Source: CAD feature listing. Evaluate the final solid. Frame: model axes, mm. Face numbers are marked on the shaded views. A direction names the side the tool comes from. Coordinates: 2 decimals unless noted, no trailing zeros. Order: outer loops, then holes, each group sorted by start corner. A loop starts at its lowest first (then second) coordinate and runs counter-clockwise, first axis right, second up.
Autodesk Inventor part; units mm, degrees
ref_plane "YZ Plane" through (0, 0, 0) normal (1, 0, 0) x (0, 1, 0)
ref_plane "XZ Plane" through (0, 0, 0) normal (0, 1, 0) x (-1, 0, 0)
ref_plane "XY Plane" through (0, 0, 0) normal (0, 0, 1) x (1, 0, 0)
sketch "Boceto1" plane through (0, 0, 0) normal (0, 1, 0) x (-1, 0, 0)
  line L0 (80, 47.68) -> (80, 52.68)
  line L1 (80, 47.68) -> (80, 22.68)
  line L2 (80, 22.68) -> (75, 22.68)
  line L3 (75, 22.68) -> (71.4886, 22.68)
  line L4 (80, 80) -> (80, 52.68)
  line L5 (20, 72.2842) -> (-29.4975, 121.7816)
  line L6 (20, 72.2842) -> (90, 72.2842) construction
  line L7 (-29.4975, 121.7816) -> (-22.4264, 128.8527)
  line L8 (29.9618, 80) -> (80, 80)
  arc A0 (71.4886, 22.68) -> (20, 72.2842) centre (0, 0) ccw
  line L9 (-22.4264, 128.8527) -> (26.4263, 80)
  line L10 (26.4263, 80) -> (29.9618, 80)
  dimension "d4" = 5
  dimension "d5" = 25
  dimension "d21" = 70
  dimension "d22" = 135
  dimension "d23" = 10
extrude "Extrusión5" add sketch "Boceto1" along normal blind 20
fillet "Empalme3" radius 80 1 edges at (-20, 10, 72.2842)
fillet "Empalme4" radius 3 4 edges at (29.4975, 10, 121.7816) (22.4264, 10, 128.8527) (-71.4886, 10, 22.68) (-80, 10, 22.68)
fillet "Empalme5" radius 30 1 edges at (-80, 10, 80)
chamfer "Chaflán1" distance 20 angle 45 1 edges at (-26.4263, 10, 80)
sketch "Boceto4" plane through (0, 20, 0) normal (0, 1, 0) x (1, 0, 0)
  arc A0 (-69.282, -40) -> (-27.3616, -75.1754) centre (0, 0) ccw
  line L0 (0, 0) -> (-69.282, -40) construction
  line L1 (0, 0) -> (80, 0) construction
  line L2 (0, 0) -> (-27.3616, -75.1754) construction
  line L3 (-69.282, -40) -> (-74.282, -40)
  line L4 (-74.282, -40) -> (-74.282, -47)
  arc A1 (-74.282, -47) -> (-27.3616, -75.1754) centre (-35.8026, -36.0762) ccw
  dimension "d35" = 80
  dimension "d36" = 150
  dimension "d37" = 40
  dimension "d38" = 5
  dimension "d39" = 7
  dimension "d40" = 40
extrude "Extrusión6" cut sketch "Boceto4" against normal blind 20
sketch "Boceto5" plane through (0, 20, 0) normal (0, 1, 0) x (1, 0, 0)
  line L0 (-80, -50) -> (-80, -25.68)
  line L1 (-46.4263, -80) -> (-50, -80)
  arc A0 (-80, -50) -> (-46.4263, -80) centre (-41.1827, -40.3452) ccw
  arc A1 (-80, -50) -> (-46.4263, -80) centre (-50.0008, -50.2137) ccw
  line L2 (-27.3616, -75.1754) -> (-17.3616, -75.1754) construction
  point P0 (0, 0)
  dimension "d43" = 40
  dimension "d44" = 30
extrude "Extrusión7" cut sketch "Boceto5" against normal blind 20
sketch "Boceto6" plane through (0, 20, 0) normal (0, 1, 0) x (1, 0, 0)
  line L0 (-36.5264, -71.1746) -> (-40.1604, -76.8501)
  line L1 (-40.1604, -76.8501) -> (-29.2954, -83.1239)
  line L2 (-29.2954, -83.1239) -> (-25.1938, -76.0206)
  line L3 (-25.1938, -76.0206) -> (-24.7057, -75.1754)
  line L4 (-24.7057, -75.1754) -> (-35.8148, -69.3243)
  line L5 (-35.8148, -69.3243) -> (-36.5264, -71.1746)
  point P0 (0, 0)
  point P1 (-74.282, -47)
  dimension "d50" = 44.8319
extrude "Extrusión8" add sketch "Boceto6" against normal blind 20
sketch "Boceto7" plane through (0, 20, 0) normal (0, 1, 0) x (1, 0, 0)
  arc A0 (-69.282, -40) -> (-36.5264, -71.1746) centre (0, 0) ccw
  line L0 (-69.282, -40) -> (-74.282, -40)
  line L1 (-69.282, -40) -> (-69.282, -40)
  arc A1 (-74.282, -47) -> (-39.5521, -75.9) centre (-35.8026, -36.0762) ccw
  line L2 (-55.1527, -57.9498) -> (-58.6667, -54.3895)
  line L3 (-66.0968, -62.1963) -> (-58.6667, -54.3895)
  line L4 (-62.599, -65.7738) -> (-55.1527, -57.9498)
  line L5 (-66.0968, -62.1963) -> (-67.4453, -63.6132)
  line L6 (-67.4453, -63.6132) -> (-64.0789, -67.3287)
  line L7 (-64.0789, -67.3287) -> (-62.599, -65.7738)
extrude "Extrusión9" add sketch "Boceto7" against normal blind 20 contours A0 L4 A1 L3 | A1 L7 L6 L5
sketch "Boceto8" plane through (-80, 0, 25.68) normal (-1, 0, 0) x (0, 0, 1)
  point P0 (-25.68, 0)
sketch "Boceto9" plane through (-80, 0, 25.68) normal (-1, 0, 0) x (0, 0, 1)
  line L0 (0, 20) -> (24.32, 20)
  line L1 (0, 0) -> (0, 20)
  line L2 (24.32, 20) -> (24.32, 0)
  line L3 (-3, 20) -> (0, 20)
  line L4 (12.16, 10) -> (22.16, 10) construction
  line L5 (19.2311, 17.0711) -> (20.9988, 15.3033)
  line L6 (19.2311, 17.0711) -> (17.4633, 18.8388)
  line L7 (5.0889, 2.9289) -> (6.8567, 1.1612)
  line L8 (5.0889, 2.9289) -> (3.3212, 4.6967)
  line L9 (3.3212, 4.6967) -> (17.4633, 18.8388)
  line L10 (20.9988, 15.3033) -> (6.8567, 1.1612)
  point P0 (-25.68, 0)
  dimension "d56" = 10
  dimension "d58" = 10
  dimension "d59" = 2.5
  dimension "d60" = 2.5
extrude "Extrusión10" add sketch "Boceto9" along normal blind 13
sketch "Boceto10" plane through (-80, 4.6967, 29.0012) normal (0, 0.7071, -0.7071) x (-1, 0, 0)
  line L0 (13, 0) -> (13, 20)
  line L1 (13, 20) -> (13, 0)
  line L2 (10, 10) -> (10, 15)
  line L3 (10, 15) -> (3, 15)
  line L4 (3, 15) -> (3, 5)
  line L5 (3, 5) -> (10, 5)
  line L6 (10, 5) -> (10, 10)
  point P0 (-80, -23.828)
  dimension "d64" = 5
  dimension "d65" = 7
  dimension "d66" = 10
extrude "Extrusión11" cut sketch "Boceto10" against normal blind 13
properties part number "Positioner_Adapter_Izq" material "ABS Plastic Black"
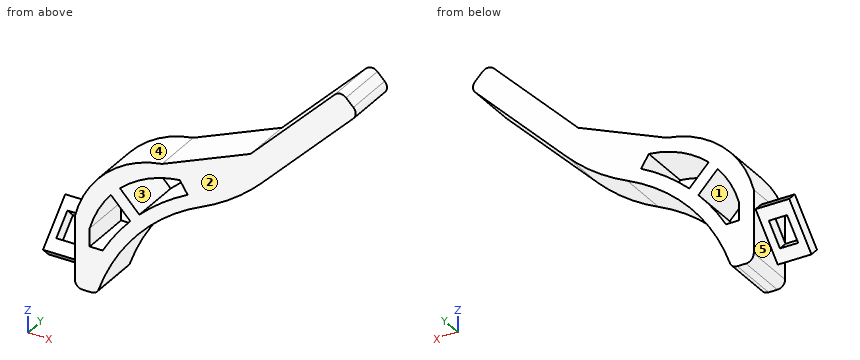
Q1. Pin query (flat end, axial travel): P1, Ø12, axis at x = -42, y = 13.5, coming from the -Z side; P2, Ø2.5, axis at x = -73, y = 5, coming from the +Z side; P3, Ø2, axis at y = 6, z = 43.5, coming from the +X side. Return the tip coordinate at first contact, or that it passes through.
Solutions:
P1: stops at z = 57.63
P2: stops at z = 66.15
P3: stops at x = -60.37
Q2. Material intervals for line 1 along Z through (x, y) = (-40.5, 7.5); line 2 along X through (y, z) = (8.5, 52); line 3 along X through (y, z) = (4.75, 57), sorted ascending.
Solutions:
line 1: z = 63.12 to 68.99, 75.8 to 82.45
line 2: x = -79.45 to -72.5, -60.79 to -54.05
line 3: x = -77.55 to -69.89, -61.15 to -48.74
Q3. Section query C-C on z = 101. Output: boundary loops of the cut face in (x, y), plus the area to 3 significant figures.
Solutions:
outline: (-5.43, 0) - (8.72, 0) - (8.72, 20) - (-5.43, 20) - close
area: 283 mm2
Q4. Section query A-A on x = -64. Output: boundary loops of the cut face in (y, z).
Solutions:
outline: (0, 39.1) - (20, 39.1) - (20, 48) - (0, 48) - close; (0, 59.99) - (20, 59.99) - (20, 73.2) - (0, 73.2) - close
Q5. Set-up query: the marked faces 1 and 2. Return all of +Z, -Z, +X, -X, +Y, -Y with unobstructed straight access to the full face (end or side cutting, diameter ignored); none if empty.
Solutions:
face 1: +Y, -Y
face 2: +Z, -Z, +X, -X, -Y
Q6. Section query B-B on y = 13.5. Give the number of separate pieces and of enclosed holes in the cut face, plus the area to 3 significant figures.
Solutions:
separate pieces: 1
enclosed holes: 2
area: 1,890 mm2
Q7. Pull-direction query (Z, two-part tool) for the marked faces 3, 4 and 5; classes: pulls with the +Z half, pulls with the -Z half, needs draft (parallel to the pull), parting line crosses it, or undercut.
Solutions:
face 3: undercut
face 4: pulls with the +Z half
face 5: needs draft
